Source: CAD feature listing. Evaluate the final solid. Frame: model axes, mm. Face numbers are marked on the shaded views. Round coordinates to 2 decimals unless told otherwise and drop trailing zeros. Order: outer loops, then holes, each group sorted by start corner. A loop starts at its lowest first (then second) coordinate and runs counter-clockwise, first axis right, second up. Notation, with made-up numbers: (43, 50.25) - (54, 50.25) arc R12 cw to (54, 60.25) - close; hole circle Ø1 at (47.5, 76). An arc over 180 degrees is marked (long way). Return JSON: item names as keys, results as strings. Group by question number.
1) Section C-C, the plane y = 23.5. Give the number of separate pieces and of enclosed holes in the cut face, plus the area to 3 significant figures.
2) Mould query, pull axis Y, two halves, no side actions, for the marked faces 1, 2 and 3. Classes: pulls with the +Y half, pulls with the -Y half, needs draft (parallel to the pull), parting line crosses it, or undercut.
3) Ray query, line 1 (X direction, y = 20, z = 3.9); line 2 (X direction, y = 30.5, z = 3.1); line 3 (Y direction, x = 18.5, z = 2.1). Return the intervals inside material, ascending. Write a range as from..to.
4) Section B-B, the plane y = 19.5. Return loops of the section in (x, z), plus the area to 3 significant figures.
5) Contact query for flat-ended pins moving along their axis: P1, Ø1, axis at x = 7, z = 2.5, coming from the -Y side; P2, Ø4.5, axis at x = 0, y = 30, coming from the +Z side; P3, Ø2, axis at x = 10.5, z = 2.5, coming from the +Y side; P4, Ø1, axis at y = 24.5, z = 4.5, coming from the -X side. Output: stop coordinate, or through.
6) Section D-D, the plane x = -13. Return loops of the section in (y, z).
7) Section A-A, the plane x = 0. Return loops of the section in (y, z), plus the area to 3 significant figures.
Autodesk Inventor part; units mm, degrees
ref_plane "YZ Plane" through (0, 0, 0) normal (1, 0, 0) x (0, 1, 0)
ref_plane "XZ Plane" through (0, 0, 0) normal (0, 1, 0) x (-1, 0, 0)
ref_plane "XY Plane" through (0, 0, 0) normal (0, 0, 1) x (1, 0, 0)
sketch "Sketch1" plane through (0, 0, 0) normal (0, 0, 1) x (1, 0, 0)
  circle A0 centre (0, 0) radius 25
  circle A1 centre (0, 0) radius 35
  line L0 (-17.6777, 17.6777) -> (-24.7487, 24.7487)
  line L1 (0, 35) -> (0, 0) construction
  line L2 (-24.0315, 25.4457) -> (-16.9564, 18.3706)
  line L3 (-1.1667, 34.9806) -> (-1.1667, 34.9972)
  line L4 (1.1667, 34.9806) -> (1.1667, 34.9972)
  line L5 (17.6777, 17.6777) -> (24.7487, 24.7487)
  line L6 (24.0315, 25.4457) -> (16.9564, 18.3706)
  line L7 (-25.4457, 24.0315) -> (-18.3706, 16.9564)
  line L8 (25.4457, 24.0315) -> (18.3706, 16.9564)
  line L9 (-1, 15) -> (1, 15)
  line L10 (1, 15) -> (1, 0)
  line L11 (1, 0) -> (-1, 0)
  line L12 (-1, 0) -> (-1, 15)
  line L13 (-1, 0) -> (1, 0)
  line L14 (1, 0) -> (1, -6)
  line L15 (1, -6) -> (-1, -6)
  line L16 (-1, -6) -> (-1, 0)
  line L17 (-1, -6) -> (-5, -6)
  line L18 (-5, -6) -> (-5, 3)
  line L19 (-5, 3) -> (-1, 3)
  line L20 (-1, 3) -> (-1, -6)
  line L21 (-5, 3) -> (-21.2192, -13.2192)
  line L22 (-5, -6) -> (-17.1706, -18.1706)
  line L23 (-5, 3) -> (-1, 15)
  line L24 (-5, -6) -> (-1, -2)
  line L25 (1, 0) -> (1, 15)
  line L26 (1, -6) -> (1, 0)
  line L27 (5, 3) -> (21.2192, -13.2192)
  line L28 (5, -6) -> (17.1706, -18.1706)
  line L29 (5, 3) -> (1, 15)
  line L30 (5, -6) -> (1, -2)
  point P0 (-20.5061, 21.9203)
  point P1 (-21.9203, 20.5061)
  point P2 (20.5061, 21.9203)
  point P3 (21.9203, 20.5061)
  point P4 (-1, -2)
  point P5 (1, 0)
  point P6 (1, -2)
  dimension "d0" = 50
  dimension "d1" = 10
  dimension "d2" = 45
  dimension "d3" = 1
  dimension "d5" = 2
  dimension "d6" = 15
  dimension "d7" = 6
  dimension "d8" = 2
  dimension "d9" = 4
  dimension "d11" = 45
  dimension "d12" = 45
  dimension "d13" = 3
  dimension "d14" = 45
extrude "Extrusion1" add sketch "Sketch1" along normal blind 5 contours A0 L2 A1 L6
sketch "Sketch3" plane through (24.0315, 25.4457, 5) normal (0.7071, -0.7071, 0) x (-0.7071, -0.7071, 0)
  line L0 (0, 5) -> (0, 0) construction
  line L1 (10.0057, 0) -> (0, 0) construction
  circle A0 centre (5.0029, 2.5) radius 1.5
  point P0 (34.9857, 5)
  dimension "d19" = 3
  dimension "d21" = 5.0029
  dimension "d22" = 2.5
extrude "Extrusion3" cut sketch "Sketch3" against normal blind 5
sketch "Sketch4" plane through (0, 0, 5) normal (0, 0, 1) x (1, 0, 0)
  arc A0 (24.0315, 25.4457) -> (-24.0315, 25.4457) centre (0, 0) ccw construction
  circle A1 centre (0, 30) radius 2.5
  point P0 (0, 35)
  dimension "d25" = 5
  dimension "d26" = 5
extrude "Extrusion4" cut sketch "Sketch4" against normal through all
mirror "Mirror1" about plane through (0, 0, 0) normal (1, 0, 0) of "Extrusion3"
properties part number "Black_Part1"
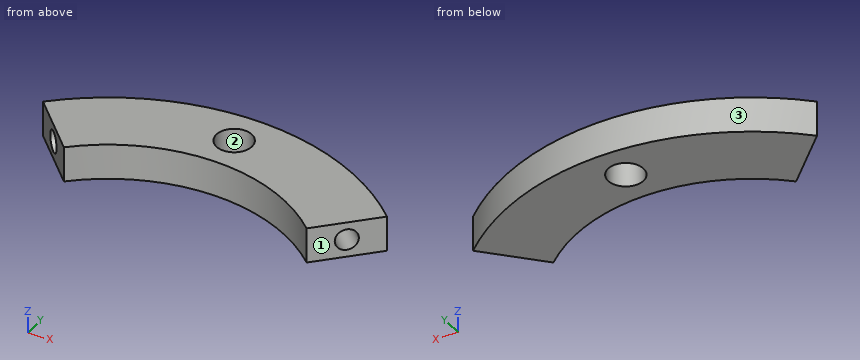
Geometry check:
{
 "1": {"separate pieces": "2", "enclosed holes": "2", "area": "116 mm2"},
 "2": {"face 1": "pulls with the -Y half", "face 2": "undercut", "face 3": "pulls with the +Y half"},
 "3": {"line 1": "-18.59..-15, 15..18.59", "line 2": "-17.17..-2.45, 2.45..17.17", "line 3": "19.91..21.86, 25.95..29.71"},
 "4": {"outline": "(-18.09, 0) - (-15.64, 0) - (-15.64, 5) - (-18.09, 5) - close; (15.64, 0) - (18.09, 0) - (18.09, 5) - (15.64, 5) - close", "area": "24.4 mm2"},
 "5": {"P1": "y = 23.85", "P2": "through", "P3": "y = 33.69", "P4": "x = -23.59"},
 "6": {"outline": "(21.35, 0) - (32.5, 0) - (32.5, 5) - (21.35, 5) - close"},
 "7": {"outline": "(25, 0) - (27.5, 0) - (27.5, 5) - (25, 5) - close; (32.5, 0) - (35, 0) - (35, 5) - (32.5, 5) - close", "area": "25.0 mm2"}
}
